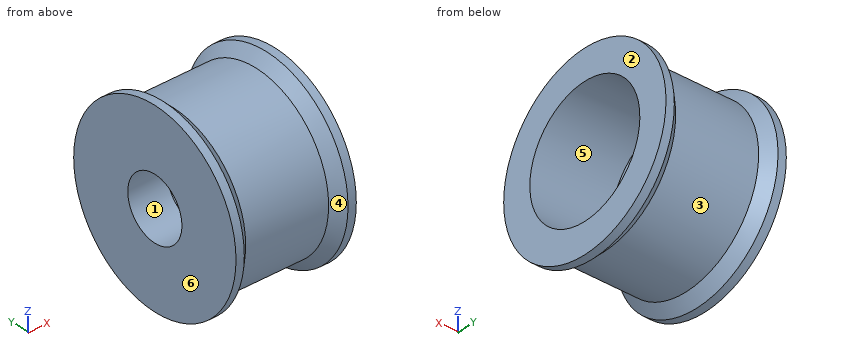
```python
from build123d import *

# Parameters (mm, degrees)
SKETCH3_R               = 3.05
CUT_EXTRUDE1_DEPTH      = 10
CUT_EXTRUDE1_DEPTH_BACK = 1


with BuildPart() as part:
    # Sketch1 → Revolve1 (revolve)
    with BuildSketch(Plane.XY):
        Polygon((-2.9, 1.5), (-2.9, 4.5), (-2.5, 4.5), (-2, 4), (2, 4), (2.5, 4.5), (2.9, 4.5), (2.9, 1.5), align=None)
    revolve(axis=Axis((0, 0, 0), (1, 0, 0)))

    # Sketch3 → Cut-Extrude1 (cut, two sides)
    with BuildSketch(Plane(origin=(0, 0, 0), x_dir=(0, 0, -1), z_dir=(1, 0, 0))) as cut_extrude1_sk:
        Circle(SKETCH3_R)
    extrude(amount=CUT_EXTRUDE1_DEPTH, mode=Mode.SUBTRACT)
    extrude(cut_extrude1_sk.sketch, amount=-CUT_EXTRUDE1_DEPTH_BACK, mode=Mode.SUBTRACT)


solid = part.part
```
Geometry check sheet. Reference: the model listing, model coordinates, mm. Face numbers are marked on the shaded views. A direction names the side the tool comes from. Give positions to 0.01 mm unless a question says otherwise; leave off trailing zeros. Write each loop counter-clockwise with the first axis right and the second up, starting at its lowest first coordinate (ties: lowest second). Pieces come first, ordered by that corner, then holes.
1) Access from +Z, -Z, +X, -X, +Y, -Y to the whole of each face (thin tool, end or side, straight path). Record for the marked faces 4, 5 and 6.
2) Section check C-C, the plane x = -2.2. Record the boundary of the cut face in (y, z), and give its area (3 significant figures).
3) Release check for a two-part mould opening along Z. For the marked faces 1, 2 and 3 record: pulls with the +Z half, pulls with the -Z half, needs draft (parallel to the pull), parting line crosses it, or undercut.
4) Material ranges on L1, parallel to Z at x = 0.1, y = 0; L2, parallel to Z at x = -1.9, y = 0; L3, parallel to X at y = 1.75, z = 2, recorded low to high.
5) Gauge pin test, flat ends, axial feed: pin 1 (2 mm diameter, centred on x = -1, z = 2.5, fed in from -Y); pin 2 (3 mm diameter, centred on y = -0.5, z = 0.5, fed in from +X); pin 3 (1 mm diameter, centred on x = -2.5, z = 2, fed in from -Y). Record the tip position at first contact, or that the pin passes through.
6) Section check A-A, the plane z = 0. Record the boundary of the cut face in (x, y).
7) Section check B-B, the plane x = 0. Record the boundary of the cut face in (y, z), and give its area (3 significant figures).
Computed:
1. face 4: none
1. face 5: +X
1. face 6: +Z, -Z, -X, +Y, -Y
2. outline: circle Ø8.4 at (0, 0); hole circle Ø3 at (0, 0)
2. area: 48.3 mm2
3. face 1: undercut
3. face 2: needs draft
3. face 3: parting line crosses it
4. L1: z = -4 to -3.05, 3.05 to 4
4. L2: z = -4 to -1.5, 1.5 to 4
4. L3: x = -2.9 to -1
5. pin 1: stops at y = -3.71
5. pin 2: stops at x = -1
5. pin 3: stops at y = -4.24
6. outline: (-2.9, -4.5) - (-2.5, -4.5) - (-2, -4) - (2, -4) - (2.5, -4.5) - (2.9, -4.5) - (2.9, -3.05) - (-1, -3.05) - (-1, -1.5) - (-2.9, -1.5) - close; (-2.9, 1.5) - (-1, 1.5) - (-1, 3.05) - (2.9, 3.05) - (2.9, 4.5) - (2.5, 4.5) - (2, 4) - (-2, 4) - (-2.5, 4.5) - (-2.9, 4.5) - close
7. outline: circle Ø8 at (0, 0); hole circle Ø6.1 at (0, 0)
7. area: 21.0 mm2
